```python
from build123d import *

# Parameters (mm, degrees)
SKETCH1_W           = 200.3
SKETCH1_H           = 200
SKETCH1_R           = 2.5
BOSS_EXTRUDE1_DEPTH = 18
FILLET1_R           = 10
SKETCH2_R           = 5
CUT_EXTRUDE1_DEPTH  = 5
SKETCH3_W           = 100
SKETCH3_H           = 150
CUT_EXTRUDE2_DEPTH  = 13
FILLET2_R           = 10
SKETCH4_R           = 5
CUT_EXTRUDE3_DEPTH  = 5
SKETCH5_R           = 2.5
CUT_EXTRUDE4_DEPTH  = 143.123265161


with BuildPart() as part:
    # Sketch1 → Boss-Extrude1 (new body)
    with BuildSketch(Plane(origin=(0, 0, 0), x_dir=(1, 0, 0), z_dir=(0, 1, 0))):
        Rectangle(SKETCH1_W, SKETCH1_H)
        with Locations(Location((86.84999973, 0, 0), (0, 0, 270))):
            Circle(SKETCH1_R, mode=Mode.SUBTRACT)
        with Locations(Location((86.84999973, 33, 0), (0, 0, 270))):
            Circle(SKETCH1_R, mode=Mode.SUBTRACT)
        with Locations(Location((86.84999973, 66, 0), (0, 0, 270))):
            Circle(SKETCH1_R, mode=Mode.SUBTRACT)
        with Locations(Location((86.84999973, -66, 0), (0, 0, 90))):
            Circle(SKETCH1_R, mode=Mode.SUBTRACT)
        with Locations(Location((86.84999973, -33, 0), (0, 0, 90))):
            Circle(SKETCH1_R, mode=Mode.SUBTRACT)
        with Locations(Location((-86.84999973, 66, 0), (0, 0, 90))):
            Circle(SKETCH1_R, mode=Mode.SUBTRACT)
        with Locations(Location((-86.84999973, 33, 0), (0, 0, 90))):
            Circle(SKETCH1_R, mode=Mode.SUBTRACT)
        with Locations(Location((-86.84999973, 0, 0), (0, 0, 90))):
            Circle(SKETCH1_R, mode=Mode.SUBTRACT)
        with Locations(Location((-86.84999973, -33, 0), (0, 0, 270))):
            Circle(SKETCH1_R, mode=Mode.SUBTRACT)
        with Locations(Location((-86.84999973, -66, 0), (0, 0, 270))):
            Circle(SKETCH1_R, mode=Mode.SUBTRACT)
        with Locations(Location((56, -60, 0), (0, 0, 270))):
            Circle(SKETCH1_R, mode=Mode.SUBTRACT)
        with Locations(Location((-56, -60, 0), (0, 0, 90))):
            Circle(SKETCH1_R, mode=Mode.SUBTRACT)
        with Locations(Location((-56, 60, 0), (0, 0, 270))):
            Circle(SKETCH1_R, mode=Mode.SUBTRACT)
        with Locations(Location((56, 60, 0), (0, 0, 90))):
            Circle(SKETCH1_R, mode=Mode.SUBTRACT)
        with BuildLine():
            Line((40, 33), (-40, 33))
            ThreePointArc((-40, 33), (-47, 40), (-40, 47))
            Line((-40, 47), (40, 47))
            ThreePointArc((40, 47), (47, 40), (40, 33))
        make_face(mode=Mode.SUBTRACT)
        with BuildLine():
            Line((40, 13), (-40, 13))
            ThreePointArc((-40, 13), (-47, 20), (-40, 27))
            Line((-40, 27), (40, 27))
            ThreePointArc((40, 27), (47, 20), (40, 13))
        make_face(mode=Mode.SUBTRACT)
        with BuildLine():
            Line((40, -7), (-40, -7))
            ThreePointArc((-40, -7), (-47, 0), (-40, 7))
            Line((-40, 7), (40, 7))
            ThreePointArc((40, 7), (47, 0), (40, -7))
        make_face(mode=Mode.SUBTRACT)
        with BuildLine():
            Line((40, -27), (-40, -27))
            ThreePointArc((-40, -27), (-47, -20), (-40, -13))
            Line((-40, -13), (40, -13))
            ThreePointArc((40, -13), (47, -20), (40, -27))
        make_face(mode=Mode.SUBTRACT)
        with BuildLine():
            Line((40, -47), (-40, -47))
            ThreePointArc((-40, -47), (-47, -40), (-40, -33))
            Line((-40, -33), (40, -33))
            ThreePointArc((40, -33), (47, -40), (40, -47))
        make_face(mode=Mode.SUBTRACT)
    extrude(amount=BOSS_EXTRUDE1_DEPTH)

    # Fillet1
    fillet1_edges = [part.edges().sort_by_distance(p)[0] for p in [
        (100.15, 9, 100),
        (-100.15, 9, 100),
        (-100.15, 9, -100),
        (100.15, 9, -100),
    ]]
    fillet(fillet1_edges, radius=FILLET1_R)

    # Sketch2 → Cut-Extrude1 (cut)
    with BuildSketch(Plane(origin=(0, 18, 0), x_dir=(1, 0, 0), z_dir=(0, 1, 0))):
        with Locations(Location((-86.84999973, 66, 0), (0, 0, 270))):
            Circle(SKETCH2_R)
        with Locations(Location((-86.84999973, 33, 0), (0, 0, 270))):
            Circle(SKETCH2_R)
        with Locations(Location((-86.84999973, 0, 0), (0, 0, 270))):
            Circle(SKETCH2_R)
        with Locations(Location((-86.84999973, -33, 0), (0, 0, 270))):
            Circle(SKETCH2_R)
        with Locations(Location((-86.84999973, -66, 0), (0, 0, 270))):
            Circle(SKETCH2_R)
        with Locations(Location((86.84999973, -66, 0), (0, 0, 90))):
            Circle(SKETCH2_R)
        with Locations(Location((86.84999973, -33, 0), (0, 0, 90))):
            Circle(SKETCH2_R)
        with Locations(Location((86.84999973, 0, 0), (0, 0, 90))):
            Circle(SKETCH2_R)
        with Locations(Location((86.84999973, 33, 0), (0, 0, 90))):
            Circle(SKETCH2_R)
        with Locations(Location((86.84999973, 66, 0), (0, 0, 90))):
            Circle(SKETCH2_R)
        with Locations(Location((-56, 60, 0), (0, 0, 270))):
            Circle(SKETCH2_R)
        with Locations(Location((-56, -60, 0), (0, 0, 90))):
            Circle(SKETCH2_R)
        with Locations(Location((56, -60, 0), (0, 0, 270))):
            Circle(SKETCH2_R)
        with Locations(Location((56, 60, 0), (0, 0, 90))):
            Circle(SKETCH2_R)
    extrude(amount=-CUT_EXTRUDE1_DEPTH, mode=Mode.SUBTRACT)

    # Sketch3 → Cut-Extrude2 (cut)
    with BuildSketch(Plane(origin=(0, 18, 0), x_dir=(1, 0, 0), z_dir=(0, 1, 0))):
        Rectangle(SKETCH3_W, SKETCH3_H)
    extrude(amount=-CUT_EXTRUDE2_DEPTH, mode=Mode.SUBTRACT)

    # Fillet2
    fillet2_edges = [part.edges().sort_by_distance(p)[0] for p in [
        (50, 11.5, -75),
        (50, 11.5, 75),
        (-50, 11.5, 75),
        (-50, 11.5, -75),
    ]]
    fillet(fillet2_edges, radius=FILLET2_R)

    # Sketch4 → Cut-Extrude3 (cut)
    with BuildSketch(Plane(origin=(0, 18, 0), x_dir=(1, 0, 0), z_dir=(0, 1, 0))):
        with Locations(Location((-90.15, -90, 0), (0, 0, 270))):
            Circle(SKETCH4_R)
        with Locations(Location((-90.15, 90, 0), (0, 0, 270))):
            Circle(SKETCH4_R)
        with Locations(Location((90.15, 90, 0), (0, 0, 270))):
            Circle(SKETCH4_R)
        with Locations(Location((90.15, -90, 0), (0, 0, 270))):
            Circle(SKETCH4_R)
    extrude(amount=-CUT_EXTRUDE3_DEPTH, mode=Mode.SUBTRACT)

    # Sketch5 → Cut-Extrude4 (cut, through all)
    with BuildSketch(Plane(origin=(0, 13, 0), x_dir=(1, 0, 0), z_dir=(0, 1, 0))):
        with Locations(Location((-90.15, -90, 0), (0, 0, 270))):
            Circle(SKETCH5_R)
        with Locations(Location((-90.15, 90, 0), (0, 0, 270))):
            Circle(SKETCH5_R)
        with Locations(Location((90.15, 90, 0), (0, 0, 270))):
            Circle(SKETCH5_R)
        with Locations(Location((90.15, -90, 0), (0, 0, 270))):
            Circle(SKETCH5_R)
    extrude(amount=-CUT_EXTRUDE4_DEPTH, mode=Mode.SUBTRACT)


solid = part.part
```
For this review, take the finished solid that the model builds, in its own axes (mm). A direction names the side the tool comes from. Coordinates: 2 decimals unless noted, no trailing zeros. Order: outer loops, then holes, each group sorted by start corner. A loop starts at its lowest first (then second) coordinate and runs counter-clockwise, first axis right, second up. Notation, with made-up numbers: (-20, 32.25) -> (4, 32.25) arc R17 cw to (4, 39.25) -> close; hole circle Ø4 at (25, 84.5). An arc over 180 degrees is marked (long way). Use CSV: the item, a comma, the result in double quotes. Start each with the question number.
Item 1: We need section B-B, the plane z = -20. Give the boundary of the cut face in (x, y), then the cut area to 3 significant figures.
Item 2: Insertion check: pin 1 (9 mm diameter, centred on x = 90.15, z = -90, fed in from +Y); pin 2 (3 mm diameter, centred on x = -56, z = 60, fed in from +Y). Each pin has a flat end and moves straight along its axis. Give the tip position at first contact, or say it passes through.
Item 3: For faces 1 (the face through (-1, 2, -7)), 2 (the face through (100.15, 9, 1)), 3 (the face through (51.043, 15.535, -59.349)), list the 3-axis set-ups (+Z, -Z, +X, -X, +Y, -Y) from which the entire face can be reached by the end or side of a thin tool; tool diameter is ignored.
Item 4: We need section A-A, the plane z = 0. Give the boundary of the cut face in (x, y).
Item 5: Draft analysis for pull direction X (two halves, no side actions). For faces 4 (the face through (-83.471, 15.535, -36.685)), 5 (the face through (97.14, 9.13, -97.15)), 6 (the face through (89.33, 6.41, -66.33)), state which applies: pulls with the +X half, pulls with the -X half, needs draft (parallel to the pull), parting line crosses it, or undercut.
Item 6: We need section C-C, the plane x = 56. Give the boundary of the cut face in (y, z), then the cut area to 3 significant figures.
Item 7: We need section D-D, the plane x = 16.5. Give the boundary of the cut face in (y, z).
Item 8: Wall thickness on probe 1 along Z at (x, y) = (86.85, 8.5); probe 2 along X at (y, z) = (14.95, 66); probe 3 along X at (y, z) = (10, -66): over which ranges is each line inside the solid? List them lowest first.
Derived:
1,outline,"(-100.15, 0) -> (-47, 0) -> (-47, 5) -> (-50, 5) -> (-50, 18) -> (-100.15, 18) -> close; (47, 0) -> (100.15, 0) -> (100.15, 18) -> (50, 18) -> (50, 5) -> (47, 5) -> close"
1,area,"1,840 mm^2"
2,pin 1,"stops at y = 13"
2,pin 2,"passes through"
3,face 1,"+Y, -Y"
3,face 2,"+Z, -Z, +X, +Y, -Y"
3,face 3,"+Y"
4,outline,"(-100.15, 0) -> (-89.35, 0) -> (-89.35, 13) -> (-91.85, 13) -> (-91.85, 18) -> (-100.15, 18) -> close; (-84.35, 0) -> (-47, 0) -> (-47, 5) -> (-50, 5) -> (-50, 18) -> (-81.85, 18) -> (-81.85, 13) -> (-84.35, 13) -> close; (47, 0) -> (84.35, 0) -> (84.35, 13) -> (81.85, 13) -> (81.85, 18) -> (50, 18) -> (50, 5) -> (47, 5) -> close; (89.35, 0) -> (100.15, 0) -> (100.15, 18) -> (91.85, 18) -> (91.85, 13) -> (89.35, 13) -> close"
5,face 4,"undercut"
5,face 5,"pulls with the +X half"
5,face 6,"undercut"
6,outline,"(0, -100) -> (18, -100) -> (18, -65) -> (13, -65) -> (13, -62.5) -> (0, -62.5) -> close; (0, -57.5) -> (13, -57.5) -> (13, -55) -> (18, -55) -> (18, 55) -> (13, 55) -> (13, 57.5) -> (0, 57.5) -> close; (0, 62.5) -> (13, 62.5) -> (13, 65) -> (18, 65) -> (18, 100) -> (0, 100) -> close"
6,area,"3,370 mm^2"
7,outline,"(0, -100) -> (18, -100) -> (18, -75) -> (5, -75) -> (5, -47) -> (0, -47) -> close; (0, -33) -> (5, -33) -> (5, -27) -> (0, -27) -> close; (0, -13) -> (5, -13) -> (5, -7) -> (0, -7) -> close; (0, 7) -> (5, 7) -> (5, 13) -> (0, 13) -> close; (0, 27) -> (5, 27) -> (5, 33) -> (0, 33) -> close; (0, 47) -> (5, 47) -> (5, 75) -> (18, 75) -> (18, 100) -> (0, 100) -> close"
8,probe 1,"z = -100 to -68.5, -63.5 to -35.5, -30.5 to -2.5, 2.5 to 30.5, 35.5 to 63.5, 68.5 to 100"
8,probe 2,"x = -100.15 to -91.85, -81.85 to -49.95, 49.95 to 81.85, 91.85 to 100.15"
8,probe 3,"x = -100.15 to -89.35, -84.35 to -49.95, 49.95 to 84.35, 89.35 to 100.15"
